from build123d import *

# Parameters (mm, degrees)
BOSS_EXTRUDE1_DEPTH = 100
CHAMFER1_SIZE       = 1.905


with BuildPart() as part:
    # Sketch3 → Boss-Extrude1 (new body)
    with BuildSketch(Plane.XY):
        with BuildLine():
            Line((-2, 3.156854249), (-2, 5.656854249))
            ThreePointArc((-2, 5.656854249), (0, -6), (2, 5.656854249))
            Line((2, 5.656854249), (2, 3.156854249))
            Line((2, 3.156854249), (-2, 3.156854249))
        make_face()
    extrude(amount=BOSS_EXTRUDE1_DEPTH)

    # Chamfer1
    chamfer1_edges = [part.edges().sort_by_distance(p)[0] for p in [
        (0, -6, 100),
        (0, -6, 0),
    ]]
    chamfer(chamfer1_edges, length=CHAMFER1_SIZE)


solid = part.part
The model under review builds one solid part; all positions refer to its coordinate system, in mm. A direction names the side the tool comes from. Give positions to 0.01 mm unless a question says otherwise; leave off trailing zeros. Write each loop counter-clockwise with the first axis right and the second up, starting at its lowest first coordinate (ties: lowest second). Pieces come first, ordered by that corner, then holes.
1. Tool access review of faces 1 (the flat face through (0, 3.157, 49)), 2 (the cylindrical face through (0, -6, 49)): name each direction out of +Z, -Z, +X, -X, +Y, -Y from which nothing blocks a thin tool from reaching the whole face with its end or side.
2. Draft analysis for pull direction X (two halves, no side actions). For faces 3 (the flat face through (-2, 4, 49)), 4 (the conical face through (-0.173, -4.396, 0.304)), 5 (the flat face through (0, 0, 0)), state which applies: +X half, -X half, draft (parallel to the pull), parting line (faces both ways), or undercut.
3. Wall thickness on L1, parallel to X at y = -0.25, z = 57.5; L2, parallel to X at y = 4.75, z = 43; L3, parallel to X at y = 4.5, z = 86: over which ranges is each line inside the solid? List them lowest first.
4. Add section B-B, the plane z = 69.5. Write out the cut boundary in (x, y), plus the area to 3 significant figures.
5. For P1, Ø2, axis at y = 4, z = 32.5, coming from the +X side; P2, Ø1.5, axis at x = 3.5, y = -4.5, coming from the +Z side; P3, Ø2, axis at x = -0.5, z = 27, coming from the +Y side; P4, Ø2, axis at x = -0.5, y = 4.5, coming from the +Z side, all flat-tipped, find the tip position at first contact; note any pin that passes through.
6. Add section A-A, the plane x = 0. Write out the cut boundary in (y, z) (3 decimals), plus the area to 3 significant figures.
Worked answers:
1. face 1: +Z, -Z, +Y
1. face 2: +Z, -Z
2. face 3: undercut
2. face 4: parting line
2. face 5: draft
3. L1: x = -5.99 to 5.99
3. L2: x = -3.67 to -2, 2 to 3.67
3. L3: x = -3.97 to -2, 2 to 3.97
4. outline: (-2, 3.16) - (-2, 5.66) arc R6 ccw (long way) to (2, 5.66) - (2, 3.16) - close
4. area: 102 mm2
5. P1: stops at x = 5.2
5. P2: stops at z = 99.14
5. P3: stops at y = 3.16
5. P4: passes through
6. outline: (-6, 1.905) - (-4.095, 0) - (3.157, 0) - (3.157, 100) - (-4.095, 100) - (-6, 98.095) - close
6. area: 912 mm2
